Can you work these out from the model? Positions are in its coordinate system, mm. Round coordinates to 2 decimals unless told otherwise and drop trailing zeros. Loops run counter-clockwise (first coordinate to the right, second up) from the corner with the lowest first, then second, coordinate; pieces in that order, holes last.
(1) I want a section at C-C on y = 0. Write out the boundary of the cut face in (x, z).
(2) Will this pin go through, and if not, where does the flat tip stop? pin 1 Ø2 at (x, y) = (6.5, 10) entering from -Z.
(3) I want a section at A-A on x = 0. Write out the boundary of the cut face in (y, z), plus the area to 3 significant figures.
(4) If I drill on line 1 along Y through (x, z) = (0, 0.5); line 2 along X through (y, z) = (-1.5, 0.75); line 3 along Y through (x, z) = (15.5, 0.1), over which ranges is the centre line in solid material (lowest first)?
(5) I want a section at D-D on x = 17. Write out the boundary of the cut face in (y, z), plus the area to 3 significant figures.
(6) I want a section at B-B on z = 0.65. Write out the boundary of the cut face in (x, y) (3 decimals).
from build123d import *

# Parameters (mm, degrees)
SKETCH1_R                   = 37.5
BOSS_EXTRUDE1_DEPTH         = 1
SKETCH2_R                   = 13
CUT_EXTRUDE1_DEPTH          = 54.042435842
TAP_DRILL_FOR_M3X0_5_TAP1_D = 3.4
CUT_EXTRUDE2_DEPTH          = 54.042435842
FILLET1_R                   = 2.5


with BuildPart() as part:
    # Sketch1 → Boss-Extrude1 (new body)
    with BuildSketch(Plane.XY):
        Circle(SKETCH1_R)
    extrude(amount=BOSS_EXTRUDE1_DEPTH)

    # Sketch2 → Cut-Extrude1 (cut, through all)
    with BuildSketch(Plane.XY.offset(1)):
        Circle(SKETCH2_R)
    extrude(amount=-CUT_EXTRUDE1_DEPTH, mode=Mode.SUBTRACT)

    # Tap Drill for M3x0.5 Tap1 (through all)
    with Locations(Plane.XY.offset(1)):
        with Locations((0, 17), (17, 0), (0, -17), (-17, 0)):
            Hole(TAP_DRILL_FOR_M3X0_5_TAP1_D / 2)

    # Sketch5 → Cut-Extrude2 (cut, through all)
    with BuildSketch(Plane.XY.offset(1)):
        with BuildLine():
            Line((27.23237189, 3.827260276), (37.135052578, 5.218991286))
            ThreePointArc((37.135052578, 5.218991286), (37.5, 0), (37.135052578, -5.218991286))
            Line((37.135052578, -5.218991286), (27.23237189, -3.827260276))
            ThreePointArc((27.23237189, -3.827260276), (27.5, 0), (27.23237189, 3.827260276))
        make_face()
    extrude(amount=-CUT_EXTRUDE2_DEPTH, mode=Mode.SUBTRACT)

    # Fillet1
    fillet1_edges = [part.edges().sort_by_distance(p)[0] for p in [
        (27.23237189, -3.827260276, 0.5),
        (27.23237189, 3.827260276, 0.5),
    ]]
    fillet(fillet1_edges, radius=FILLET1_R)


solid = part.part
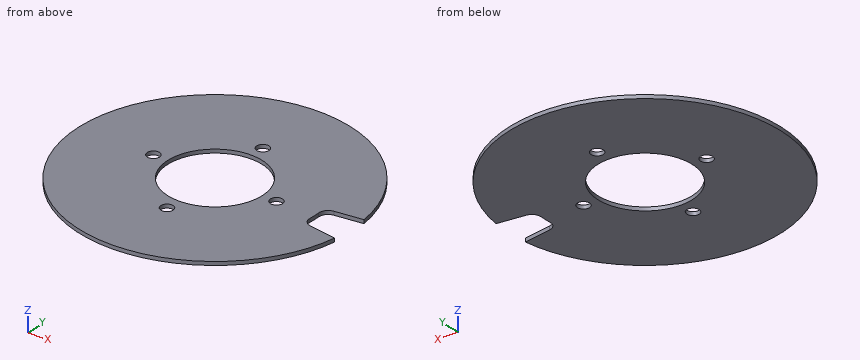
Filled sheet:
1. outline: (-37.5, 0) - (-18.7, 0) - (-18.7, 1) - (-37.5, 1) - close; (-15.3, 0) - (-13, 0) - (-13, 1) - (-15.3, 1) - close; (13, 0) - (15.3, 0) - (15.3, 1) - (13, 1) - close; (18.7, 0) - (27.5, 0) - (27.5, 1) - (18.7, 1) - close
2. pin 1: passes through
3. outline: (-37.5, 0) - (-18.7, 0) - (-18.7, 1) - (-37.5, 1) - close; (-15.3, 0) - (-13, 0) - (-13, 1) - (-15.3, 1) - close; (13, 0) - (15.3, 0) - (15.3, 1) - (13, 1) - close; (18.7, 0) - (37.5, 0) - (37.5, 1) - (18.7, 1) - close
3. area: 42.2 mm2
4. line 1: y = -37.5 to -18.7, -15.3 to -13, 13 to 15.3, 18.7 to 37.5
4. line 2: x = -37.47 to -17.8, -16.2 to -12.91, 12.91 to 16.2, 17.8 to 27.46
4. line 3: y = -34.15 to -0.8, 0.8 to 34.15
5. outline: (-33.43, 0) - (-1.7, 0) - (-1.7, 1) - (-33.43, 1) - close; (1.7, 0) - (33.43, 0) - (33.43, 1) - (1.7, 1) - close
5. area: 63.5 mm2
6. outline: (27.457, -1.545) arc R27.5 ccw to (27.457, 1.545) arc R2.5 cw to (29.605, 4.161) - (37.135, 5.219) arc R37.5 ccw (long way) to (37.135, -5.219) - (29.605, -4.161) arc R2.5 cw to start; hole circle Ø3.4 at (-17, 0); hole circle Ø26 at (0, 0); hole circle Ø3.4 at (0, -17); hole circle Ø3.4 at (0, 17); hole circle Ø3.4 at (17, 0)
